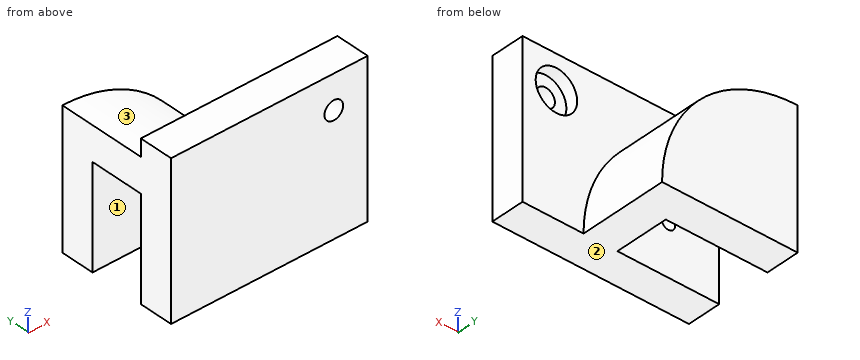
```python
from build123d import *

# Parameters (mm, degrees)
SKETCH3_W                               = 58
SKETCH3_H                               = 45
BOSS_EXTRUDE1_DEPTH                     = 10
CBORE_FOR_M5_HEX_HEAD_BOLT1_D           = 5.5
CBORE_FOR_M5_HEX_HEAD_BOLT1_CBORE_D     = 12.24
CBORE_FOR_M5_HEX_HEAD_BOLT1_CBORE_DEPTH = 3.58
BOSS_EXTRUDE3_DEPTH                     = 16
BOSS_EXTRUDE4_DEPTH                     = 10
SKETCH10_R                              = 2
CUT_EXTRUDE2_DEPTH                      = 6


with BuildPart() as part:
    # Sketch3 → Boss-Extrude1 (new body)
    with BuildSketch(Plane(origin=(0, 0, 0), x_dir=(1, 0, 0), z_dir=(0, 1, 0))):
        Rectangle(SKETCH3_W, SKETCH3_H)
    extrude(amount=BOSS_EXTRUDE1_DEPTH)

    # CBORE for M5 Hex Head Bolt1 (through all)
    with Locations(Plane(origin=(0, 10, 0), x_dir=(1, 0, 0), z_dir=(0, 1, 0))):
        with Locations((19, -12.5)):
            CounterBoreHole(CBORE_FOR_M5_HEX_HEAD_BOLT1_D / 2, CBORE_FOR_M5_HEX_HEAD_BOLT1_CBORE_D / 2, CBORE_FOR_M5_HEX_HEAD_BOLT1_CBORE_DEPTH)

    # Sketch8 → Boss-Extrude3 (add)
    with BuildSketch(Plane(origin=(0, 10, 0), x_dir=(1, 0, 0), z_dir=(0, 1, 0))):
        with BuildLine():
            Line((11, 22.5), (1, 22.5))
            ThreePointArc((1, 22.5), (-7.786796564, 1.286796564), (-29, -7.5))
            Line((-29, -7.5), (-29, -17.5))
            ThreePointArc((-29, -17.5), (-0.715728753, -5.784271247), (11, 22.5))
        make_face()
    extrude(amount=BOSS_EXTRUDE3_DEPTH)

    # Sketch9 → Boss-Extrude4 (add)
    with BuildSketch(Plane(origin=(0, 26, 0), x_dir=(1, 0, 0), z_dir=(0, 1, 0))):
        with BuildLine():
            Line((11, 22.5), (-29, 22.5))
            Line((-29, 22.5), (-29, -17.5))
            ThreePointArc((-29, -17.5), (-0.715728753, -5.784271247), (11, 22.5))
        make_face()
    extrude(amount=BOSS_EXTRUDE4_DEPTH)

    # Sketch10 → Cut-Extrude2 (cut)
    with BuildSketch(Plane(origin=(0, 10, 0), x_dir=(1, 0, 0), z_dir=(0, 1, 0))):
        with Locations(Location((-14, 7.5, 0), (0, 0, 270))):
            Circle(SKETCH10_R)
    extrude(amount=-CUT_EXTRUDE2_DEPTH, mode=Mode.SUBTRACT)


solid = part.part
```
The listing builds one solid part. Answer for the finished solid, in the listing's coordinates (mm). Face numbers are marked on the shaded views. A direction names the side the tool comes from. Give positions to 0.01 mm unless a question says otherwise; leave off trailing zeros. Order: outer loops, then holes, each group sorted by start corner. A loop starts at its lowest first (then second) coordinate and runs counter-clockwise, first axis right, second up.
Item 1: Which of the six approach directions +Z, -Z, +X, -X, +Y, -Y give full straight-line access (tool end or side, diameter ignored) to the marked faces 1, 2 and 3?
From the geometry:
face 1: -Z, -X
face 2: -Z, +X, -X, +Y, -Y
face 3: +Z, +X, +Y
Item 2: Find the intervals of material crossed by probe 1 along X at (y, z) = (4, 12.5); probe 2 along Z at (x, y) = (19, 5); probe 3 along Y at (x, z) = (22.5, 19), in increasing order.
From the geometry:
probe 1: x = -29 to 16.25, 21.75 to 29
probe 2: z = -22.5 to 9.75, 15.25 to 22.5
probe 3: y = 0 to 10
Item 3: The part is cut by section B-B, the plane y = 8.5. Give the vertices of the cut face in (x, z).
From the geometry:
outline: (-29, -22.5) - (29, -22.5) - (29, 22.5) - (-29, 22.5) - close; hole circle Ø4 at (-14, -7.5); hole circle Ø12.24 at (19, 12.5)
Item 4: The part is cut by section A-A, the plane x = 19. Give the vertices of the cut face in (y, z).
From the geometry:
outline: (0, -22.5) - (10, -22.5) - (10, 6.38) - (6.42, 6.38) - (6.42, 9.75) - (0, 9.75) - close; (0, 15.25) - (6.42, 15.25) - (6.42, 18.62) - (10, 18.62) - (10, 22.5) - (0, 22.5) - close
Item 5: Given pin 1 Ø6 at (x, y) = (-9, 16) entering from -Z; pin 2 Ø2 at (x, y) = (-12.5, 18) entering from -Z; pin 3 Ø1.5 at (x, y) = (-21, 11) entering from -Z, each flat-ended and moving along its own axis, determine where each tip first touches the part or whether it passes through.
From the geometry:
pin 1: stops at z = -3.24
pin 2: stops at z = 1.87
pin 3: stops at z = 6.2
Item 6: The part is cut by section D-D, the plane x = 6. Give the vertices of the cut face in (y, z).
From the geometry:
outline: (0, -22.5) - (36, -22.5) - (36, -3.14) - (10, -3.14) - (10, 22.5) - (0, 22.5) - close
Item 7: The part is cut by section C-C, the plane z = 19.5. Give the vertices of the cut face in (x, y), and give its area (3 significant figures).
From the geometry:
outline: (-29, 0) - (29, 0) - (29, 10) - (-29, 10) - close
area: 580 mm2
